```python
from build123d import *

# Parameters (mm, degrees)
SKETCH1_W           = 304.8
SKETCH1_H           = 38.1
BOSS_EXTRUDE5_DEPTH = 38.1
BOSS_EXTRUDE6_DEPTH = 25.4
BOSS_EXTRUDE7_DEPTH = 25.4
BOSS_EXTRUDE8_DEPTH = 482.6


with BuildPart() as part:
    # Sketch1 → Boss-Extrude5 (new body)
    with BuildSketch(Plane(origin=(0, 0, 0), x_dir=(0, 0, -1), z_dir=(1, 0, 0))):
        with Locations((0, 19.05)):
            Rectangle(SKETCH1_W, SKETCH1_H)
    extrude(amount=BOSS_EXTRUDE5_DEPTH)

    # Sketch7 → Boss-Extrude6 (add)
    with BuildSketch(Plane.XY.offset(152.4)):
        with BuildLine():
            ThreePointArc((28.011830747, 28.011830747), (19.05, 31.723942586), (10.088169253, 28.011830747))
            Line((10.088169253, 28.011830747), (19.05, 19.05))
            Line((19.05, 19.05), (28.011830747, 28.011830747))
        make_face()
        with BuildLine():
            Line((19.05, 19.05), (10.088169253, 28.011830747))
            ThreePointArc((10.088169253, 28.011830747), (6.376057414, 19.05), (10.088169253, 10.088169253))
            Line((10.088169253, 10.088169253), (19.05, 19.05))
        make_face()
        with BuildLine():
            Line((28.011830747, 28.011830747), (19.05, 19.05))
            Line((19.05, 19.05), (28.011830747, 10.088169253))
            ThreePointArc((28.011830747, 10.088169253), (30.759196151, 14.19989215), (31.723942586, 19.05))
            ThreePointArc((31.723942586, 19.05), (30.759196151, 23.90010785), (28.011830747, 28.011830747))
        make_face()
        with BuildLine():
            Line((28.011830747, 10.088169253), (19.05, 19.05))
            Line((19.05, 19.05), (10.088169253, 10.088169253))
            ThreePointArc((10.088169253, 10.088169253), (19.05, 6.376057414), (28.011830747, 10.088169253))
        make_face()
    extrude(amount=BOSS_EXTRUDE6_DEPTH)

    # Sketch8 → Boss-Extrude7 (add)
    with BuildSketch(Plane(origin=(0, 0, -152.4), x_dir=(-1, 0, 0), z_dir=(0, 0, -1))):
        with BuildLine():
            ThreePointArc((-10.044344025, 28.055655975), (-19.05, 31.785920818), (-28.055655975, 28.055655975))
            Line((-28.055655975, 28.055655975), (-19.05, 19.05))
            Line((-19.05, 19.05), (-10.044344025, 28.055655975))
        make_face()
        with BuildLine():
            Line((-19.05, 19.05), (-28.055655975, 28.055655975))
            ThreePointArc((-28.055655975, 28.055655975), (-31.785920818, 19.05), (-28.055655975, 10.044344025))
            Line((-28.055655975, 10.044344025), (-19.05, 19.05))
        make_face()
        with BuildLine():
            Line((-10.044344025, 28.055655975), (-19.05, 19.05))
            Line((-19.05, 19.05), (-10.044344025, 10.044344025))
            ThreePointArc((-10.044344025, 10.044344025), (-7.283543428, 14.176174107), (-6.314079182, 19.05))
            ThreePointArc((-6.314079182, 19.05), (-7.283543428, 23.923825893), (-10.044344025, 28.055655975))
        make_face()
        with BuildLine():
            Line((-10.044344025, 10.044344025), (-19.05, 19.05))
            Line((-19.05, 19.05), (-28.055655975, 10.044344025))
            ThreePointArc((-28.055655975, 10.044344025), (-19.05, 6.314079182), (-10.044344025, 10.044344025))
        make_face()
    extrude(amount=BOSS_EXTRUDE7_DEPTH)

    # Sketch9 → Boss-Extrude8 (add)
    with BuildSketch(Plane(origin=(38.1, 0, 0), x_dir=(0, 0, -1), z_dir=(1, 0, 0))):
        with BuildLine():
            Line((-16.624944564, 0), (0, 0))
            Line((0, 0), (0, 38.1))
            Line((0, 38.1), (-16.624944564, 38.1))
            ThreePointArc((-16.624944564, 38.1), (-25.284210127, 19.05), (-16.624944564, 0))
        make_face()
        with BuildLine():
            Line((0, 38.1), (0, 0))
            Line((0, 0), (16.624944564, 0))
            ThreePointArc((16.624944564, 0), (23.01781781, 8.587144509), (25.284210127, 19.05))
            ThreePointArc((25.284210127, 19.05), (23.01781781, 29.512855491), (16.624944564, 38.1))
            Line((16.624944564, 38.1), (0, 38.1))
        make_face()
    extrude(amount=BOSS_EXTRUDE8_DEPTH)


solid = part.part
```
Verification items for the finished model (mm, model axes). A direction names the side the tool comes from. Round coordinates to 2 decimals unless told otherwise and drop trailing zeros. Write each loop counter-clockwise with the first axis right and the second up, starting at its lowest first coordinate (ties: lowest second). Pieces come first, ordered by that corner, then holes. Notation, with made-up numbers: (20, 9.5) -> (78, 9.5) arc R22 cw to (78, 27.5) -> close; hole circle Ø2 at (26, -40). An arc over 180 degrees is marked (long way). Write each question's results on one line, items separated by ' | '. Start each with the question number.
1. Material ranges on probe 1 along X at (y, z) = (5.5, -132); probe 2 along Y at (x, z) = (466, 19); probe 3 along Z at (x, y) = (325, 12), recorded low to high. Write a range as from..to.
2. Cross-section at B-B (z = -41.5). Enter the section's corners in (x, y).
3. Cross-section at A-A (x = 313.5). Enter the section's corners in (y, z).
4. Set-up check for faces 1 (the flat face through (19, 6, 152.4)), 2 (the cylindrical face through (276.022, 19.352, 25.282)), 3 (the flat face through (19, 6, -152.4)): record each of +Z, -Z, +X, -X, +Y, -Y from which the full face is reachable in a straight line by a thin tool's end or side.
5. Depth check by flat-ended pin: P1, Ø6, axis at x = 381, y = 30, coming from the +Z side; P2, Ø5, axis at x = 411.5, y = 33, coming from the -Z side; P3, Ø5, axis at x = 160, z = 23, coming from the +Y side. Enter the tip coordinate at first touch or a pass-through.
Solutions:
1) probe 1: x = 0..38.1 | probe 2: y = 2.37..35.73 | probe 3: z = -24.28..24.28
2) outline: (0, 0) -> (38.1, 0) -> (38.1, 38.1) -> (0, 38.1) -> close
3) outline: (0, -16.62) arc R25.28 ccw to (38.1, -16.62) -> (38.1, 16.62) arc R25.28 ccw to (0, 16.62) -> close
4) face 1: +Z | face 2: +Z, +X | face 3: -Z
5) P1: stops at z = 24 | P2: stops at z = -22.54 | P3: stops at y = 33.85
